Verification items for the finished model (mm, model axes). Give positions to 0.01 mm unless a question says otherwise; leave off trailing zeros. Loops run counter-clockwise (first coordinate to the right, second up) from the corner with the lowest first, then second, coordinate; pieces in that order, holes last. Notation, with made-up numbers: (-17.75, 29.5) - (28.25, 29.5) arc R33 ccw to (28.25, 62.5) - close; hole circle Ø6 at (52, 41.25). An arc over 180 degrees is marked (long way). One line per item, written item: value. Start each with the question number.
1. Gauge pin test, flat end, axial feed: pin 1 (5 mm diameter, centred on x = 0, z = 203.2, fed in from -Y). Record the tip position at first contact, or that the pin passes through.
2. Scan lines: L1, parallel to Z at x = 203.2, y = 3.35; L2, parallel to X at y = 1.65, z = -184.15 (3 decimals). Record each from-to range of solid material in increasing order. Write a range as [from, to].
3. Sectioned sample at A-A (x = 69.85). Record the cut outline in (y, z).
from build123d import *

# Parameters (mm, degrees)
SKETCH1_W           = 457.2
SKETCH1_H           = 457.2
BOSS_EXTRUDE1_DEPTH = 4.826
SKETCH2_R           = 7.62
SKETCH2_R_2         = 6.35
CUT_EXTRUDE1_DEPTH  = 25.4
SKETCH4_R           = 3.175
CUT_EXTRUDE2_DEPTH  = 5.08
SKETCH6_R           = 3.2639
CUT_EXTRUDE3_DEPTH  = 12.7
SKETCH8_R           = 3.175
CUT_EXTRUDE5_DEPTH  = 5.826


with BuildPart() as part:
    # Sketch1 → Boss-Extrude1 (new body)
    with BuildSketch(Plane(origin=(0, 0, 0), x_dir=(1, 0, 0), z_dir=(0, 1, 0))):
        Rectangle(SKETCH1_W, SKETCH1_H)
    extrude(amount=BOSS_EXTRUDE1_DEPTH)

    # Sketch2 → Cut-Extrude1 (cut)
    with BuildSketch(Plane(origin=(0, 4.826, 0), x_dir=(1, 0, 0), z_dir=(0, 1, 0))):
        with Locations((69.85, 50.8)):
            Circle(SKETCH2_R)
        with Locations((-69.85, 50.8)):
            Circle(SKETCH2_R)
        with Locations((0, -38.1)):
            Circle(SKETCH2_R_2)
    extrude(amount=-CUT_EXTRUDE1_DEPTH, mode=Mode.SUBTRACT)

    # Sketch4 → Cut-Extrude2 (cut)
    with BuildSketch(Plane(origin=(0, 4.826, 0), x_dir=(1, 0, 0), z_dir=(0, 1, 0))):
        with Locations((-184.15, 184.15)):
            Circle(SKETCH4_R)
        with Locations((184.15, 184.15)):
            Circle(SKETCH4_R)
        with Locations((184.15, -184.15)):
            Circle(SKETCH4_R)
        with Locations((-184.15, -184.15)):
            Circle(SKETCH4_R)
    extrude(amount=-CUT_EXTRUDE2_DEPTH, mode=Mode.SUBTRACT)

    # Sketch6 → Cut-Extrude3 (cut)
    with BuildSketch(Plane(origin=(0, 4.826, 0), x_dir=(1, 0, 0), z_dir=(0, 1, 0))):
        with Locations((203.2, -203.2)):
            Circle(SKETCH6_R)
        with Locations((-203.2, 203.2)):
            Circle(SKETCH6_R)
        with Locations((203.2, -101.6)):
            Circle(SKETCH6_R)
        with Locations((203.2, 0)):
            Circle(SKETCH6_R)
        with Locations((203.2, 101.6)):
            Circle(SKETCH6_R)
        with Locations((203.2, 203.2)):
            Circle(SKETCH6_R)
        with Locations((101.6, -203.2)):
            Circle(SKETCH6_R)
        with Locations((0, -203.2)):
            Circle(SKETCH6_R)
        with Locations((-101.6, -203.2)):
            Circle(SKETCH6_R)
        with Locations((-203.2, -203.2)):
            Circle(SKETCH6_R)
        with Locations((304.8, -203.2)):
            Circle(SKETCH6_R)
        with Locations((-101.6, 203.2)):
            Circle(SKETCH6_R)
        with Locations((406.4, -203.2)):
            Circle(SKETCH6_R)
        with Locations((0, 203.2)):
            Circle(SKETCH6_R)
        with Locations((508, -203.2)):
            Circle(SKETCH6_R)
        with Locations((101.6, 203.2)):
            Circle(SKETCH6_R)
        with Locations((203.2, -304.8)):
            Circle(SKETCH6_R)
        with Locations((-203.2, 101.6)):
            Circle(SKETCH6_R)
        with Locations((203.2, -406.4)):
            Circle(SKETCH6_R)
        with Locations((-203.2, 0)):
            Circle(SKETCH6_R)
        with Locations((203.2, -508)):
            Circle(SKETCH6_R)
        with Locations((-203.2, -101.6)):
            Circle(SKETCH6_R)
    extrude(amount=-CUT_EXTRUDE3_DEPTH, mode=Mode.SUBTRACT)

    # Sketch8 → Cut-Extrude5 (cut, through all)
    with BuildSketch(Plane(origin=(0, 4.826, 0), x_dir=(1, 0, 0), z_dir=(0, 1, 0))):
        with Locations((-101.6, 50.8)):
            Circle(SKETCH8_R)
        with Locations((-38.1, 50.8)):
            Circle(SKETCH8_R)
        with Locations((38.1, 50.8)):
            Circle(SKETCH8_R)
        with Locations((101.6, 50.8)):
            Circle(SKETCH8_R)
    extrude(amount=-CUT_EXTRUDE5_DEPTH, mode=Mode.SUBTRACT)


solid = part.part
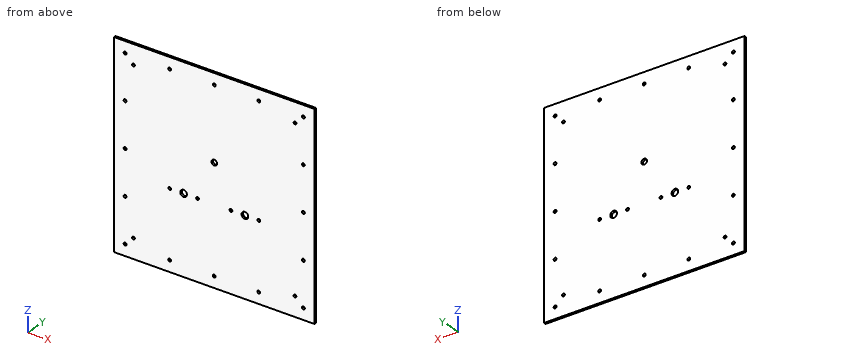
Results are:
1. pin 1: passes through
2. L1: z = [-228.6, -206.46], [-199.94, -104.86], [-98.34, -3.26], [3.26, 98.34], [104.86, 199.94], [206.46, 228.6]
2. L2: x = [-228.6, -187.325], [-180.975, 180.975], [187.325, 228.6]
3. outline: (0, -228.6) - (4.83, -228.6) - (4.83, -58.42) - (0, -58.42) - close; (0, -43.18) - (4.83, -43.18) - (4.83, 228.6) - (0, 228.6) - close
